Input: part model. Units: mm. Frame: model coordinates. Face numbers are marked on the shaded views. A direction names the side the tool comes from. Give positions to 0.01 mm unless a question says otherwise; leave off trailing zeros. Loops run counter-clockwise (first coordinate to the right, second up) from the corner with the lowest first, then second, coordinate; pieces in that order, holes last. Notation, with made-up numbers: (-27.75, 19.5) - (21.25, 19.5) arc R12 ccw to (21.25, 25.5) - close; hole circle Ø4 at (15, 70.5). An arc over 180 degrees is marked (long way). One line per item, written item: value.
from build123d import *

# Parameters (mm, degrees)
SKETCH002_R     = 2
PAD003_DEPTH    = 12
SKETCH003_R     = 0.75
PAD004_DEPTH    = 0.75
CHAMFER001_SIZE = 0.5


with BuildPart() as part:
    # Sketch002 → Pad003 (new body)
    with BuildSketch(Plane.XY):
        Circle(SKETCH002_R)
    extrude(amount=PAD003_DEPTH)

    # Sketch003 (on Face3 of Pad003) → Pad004 (join)
    with BuildSketch(Plane.XY.offset(12)):
        Circle(SKETCH003_R)
    extrude(amount=PAD004_DEPTH)

    # Chamfer001
    chamfer001_edges = [part.edges().sort_by_distance(p)[0] for p in [
        (-0.75, 0, 12.75),
    ]]
    chamfer(chamfer001_edges, length=CHAMFER001_SIZE)


solid = part.part
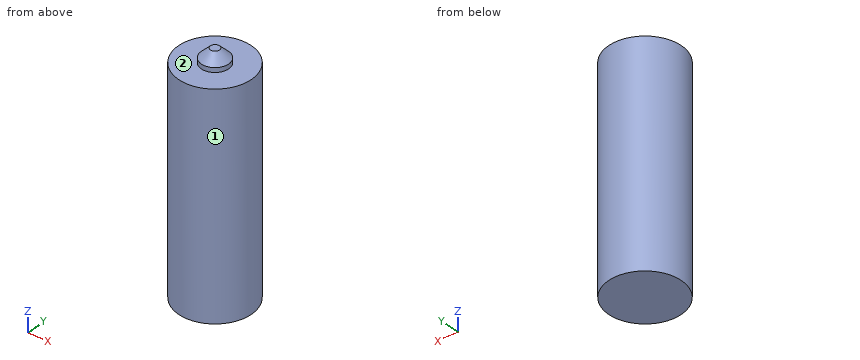
Item 1: Access query for the marked faces 1 and 2. Directions: +Z, -Z, +X, -X, +Y, -Y. A direction counts if a zero-diameter tool reaches every point of the face in a straight line with its end or side. Return the directions, or none.
Verdict:
face 1: +Z, -Z
face 2: +Z
Item 2: Material intervals for L1, parallel to Z at x = 0.4, y = -0.9; L2, parallel to X at y = -0.2, z = 2.75; L3, parallel to Y at x = 0.35, z = 8.75, sorted ascending.
Verdict:
L1: z = 0 to 12
L2: x = -1.99 to 1.99
L3: y = -1.97 to 1.97
Item 3: Section D-D, the plane x = -1.45. Output: boundary loops of the cut face in (y, z).
Verdict:
outline: (-1.38, 0) - (1.38, 0) - (1.38, 12) - (-1.38, 12) - close
Item 4: Pin query (flat end, axial travel): P1, Ø1.5, axis at y = 1, z = 2, coming from the +X side; P2, Ø1, axis at x = 1, z = 2.5, coming from the -Y side. Return the tip coordinate at first contact, or that it passes through.
Verdict:
P1: stops at x = 1.98
P2: stops at y = -1.94
Item 5: Section C-C, the plane z = 10.25. Output: boundary loops of the cut face in (x, y).
Verdict:
outline: circle Ø4 at (0, 0)
Item 6: Section A-A, the plane y = 0. Output: boundary loops of the cut face in (x, z), and give its area (3 significant figures).
Verdict:
outline: (-2, 0) - (2, 0) - (2, 12) - (0.75, 12) - (0.75, 12.25) - (0.25, 12.75) - (-0.25, 12.75) - (-0.75, 12.25) - (-0.75, 12) - (-2, 12) - close
area: 48.9 mm^2
